from build123d import *

# Parameters (mm, degrees)
BOSS_EXTRUDE1_DEPTH = 15
CUT_EXTRUDE1_DEPTH  = 23.005681085
FILLET1_R           = 0.5


with BuildPart() as part:
    # Sketch1 → Boss-Extrude1 (new body)
    with BuildSketch(Plane.XY):
        with BuildLine():
            Line((0, 0), (0, 11))
            ThreePointArc((0, 11), (3.5, 14.5), (7, 11))
            Line((7, 11), (7, 0))
            ThreePointArc((7, 0), (3.5, -3.5), (0, 0))
        make_face()
    extrude(amount=BOSS_EXTRUDE1_DEPTH)

    # Sketch2 → Cut-Extrude1 (cut, through all)
    with BuildSketch(Plane.XY.offset(15)):
        with BuildLine():
            Line((6, 0), (6, 11))
            ThreePointArc((6, 11), (3.5, 13.5), (1, 11))
            Line((1, 11), (1, 0))
            ThreePointArc((1, 0), (3.5, -2.5), (6, 0))
        make_face()
    extrude(amount=-CUT_EXTRUDE1_DEPTH, mode=Mode.SUBTRACT)

    # Fillet1
    fillet1_edges = [part.edges().sort_by_distance(p)[0] for p in [
        (3.5, -2.5, 0),
        (1, 5.5, 0),
        (3.5, 13.5, 0),
        (6, 5.5, 0),
        (3.5, -2.5, 15),
        (6, 5.5, 15),
        (3.5, 13.5, 15),
        (1, 5.5, 15),
    ]]
    fillet(fillet1_edges, radius=FILLET1_R)


solid = part.part
Model file for the job. Use its own axes, mm. A direction names the side the tool comes from. Round coordinates to 2 decimals unless told otherwise and drop trailing zeros. Order: outer loops, then holes, each group sorted by start corner. A loop starts at its lowest first (then second) coordinate and runs counter-clockwise, first axis right, second up.
(1) Band-saw the part on B-B (x = 3.5). List the corners of the cut face in (y, z), then the cut area to 3 significant figures.
(2) 3-axis set-ups, long thin cutter, end or side, ignore diameter. For faces 5 (the face through (3.6, -3.5, 7.4)), 6 (the face through (3.6, 13.5, 7.6)): which of +Z, -Z, +X, -X, +Y, -Y reach the whole face in a straight line?
(3) Band-saw the part on C-C (z = 6.75). List the corners of the cut face in (x, y).
(4) Pull direction X, two halves, no side cores. Call faces 1 (the face through (0, 5, 7)), 2 (the face through (6, 5, 8)), 3 (the face through (3.4, 14.5, 7.4)), 4 (the face through (7, 6, 7)): released by +X, released by -X, zero draft, split by the parting line, or undercut.
(5) Drill centre lines: line 1 (X direction, y = 6.5, z = 7.25); line 2 (Y direction, x = 2.5, z = 13); line 3 (X direction, y = 13, z = 6.25). Where is each one in solid material? Low to high.
(6) Band-saw the part on A-A (y = 4.5). List the corners of the cut face in (x, z), then the cut area to 3 significant figures.
(7) Pin check, flat tip, straight feed: pin 1 (3.5 mm diameter, centred on y = 3.5, z = 11, fed in from -X). Stop position of the tip, or through.
Verdict:
1. outline: (-3.5, 0) - (-3, 0) arc R0.5 ccw to (-2.5, 0.5) - (-2.5, 14.5) arc R0.5 ccw to (-3, 15) - (-3.5, 15) - close; (13.5, 0.5) arc R0.5 ccw to (14, 0) - (14.5, 0) - (14.5, 15) - (14, 15) arc R0.5 ccw to (13.5, 14.5) - close
1. area: 29.8 mm2
2. face 5: +Z, -Z, -Y
2. face 6: +Z, -Z
3. outline: (0, 0) arc R3.5 ccw to (7, 0) - (7, 11) arc R3.5 ccw to (0, 11) - close; hole (1, 0) arc R2.5 ccw to (6, 0) - (6, 11) arc R2.5 ccw to (1, 11) - close
4. face 1: released by -X
4. face 2: undercut
4. face 3: split by the parting line
4. face 4: released by +X
5. line 1: x = 0 to 1, 6 to 7
5. line 2: y = -3.35 to -2.29, 13.29 to 14.35
5. line 3: x = 0.63 to 2, 5 to 6.37
6. outline: (0, 0) - (0.5, 0) arc R0.5 ccw to (1, 0.5) - (1, 14.5) arc R0.5 ccw to (0.5, 15) - (0, 15) - close; (6, 0.5) arc R0.5 ccw to (6.5, 0) - (7, 0) - (7, 15) - (6.5, 15) arc R0.5 ccw to (6, 14.5) - close
6. area: 29.8 mm2
7. pin 1: stops at x = 0
